from build123d import *

# Parameters (mm, degrees)
BOSS_EXTRUDE1_DEPTH = 2.0574
SKETCH2_R           = 2.54
BOSS_EXTRUDE2_DEPTH = 14.605
FILLET1_R           = 0.635


with BuildPart() as part:
    # Sketch1 → Boss-Extrude1 (new, symmetric)
    with BuildSketch(Plane(origin=(0, 0, 0), x_dir=(1, 0, 0), z_dir=(0, 1, 0))):
        Polygon((-2.7305, -1.57645491), (0, -3.15290982), (2.7305, -1.57645491), (2.7305, 1.57645491), (0, 3.15290982), (-2.7305, 1.57645491), align=None)
    extrude(amount=BOSS_EXTRUDE1_DEPTH, both=True)

    # Sketch2 → Boss-Extrude2 (add)
    with BuildSketch(Plane(origin=(0, 2.0574, 0), x_dir=(1, 0, 0), z_dir=(0, 1, 0))):
        with Locations(Location((0, 0, 0), (0, 0, 90))):
            Circle(SKETCH2_R)
    boss_extrude2 = extrude(amount=BOSS_EXTRUDE2_DEPTH)

    # Mirror1: Boss-Extrude2 across plane
    add(boss_extrude2.mirror(Plane.ZX))

    # Fillet1
    fillet1_edges = [part.edges().sort_by_distance(p)[0] for p in [
        (0, 16.6624, 2.54),
        (0, -16.6624, 2.54),
    ]]
    fillet(fillet1_edges, radius=FILLET1_R)


solid = part.part
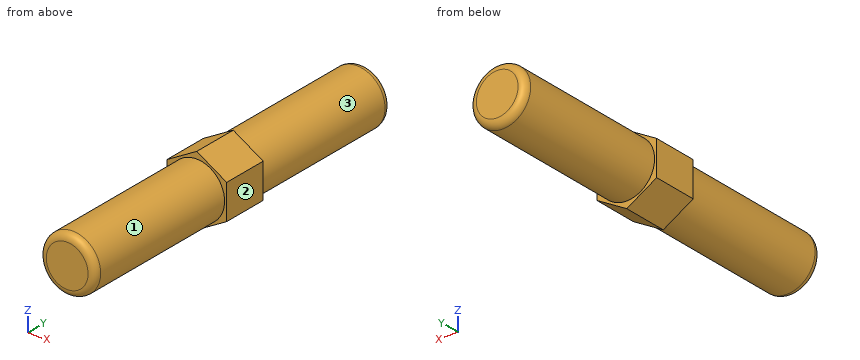
Input: part model. Units: mm. Frame: model coordinates. Face numbers are marked on the shaded views. A direction names the side the tool comes from. Round coordinates to 2 decimals unless told otherwise and drop trailing zeros. Order: outer loops, then holes, each group sorted by start corner. A loop starts at its lowest first (then second) coordinate and runs counter-clockwise, first axis right, second up. Notation, with made-up numbers: (86.5, -31.5) - (120.5, -31.5) arc R30 ccw to (120.5, -9.5) - close; hole circle Ø8 at (69, 30.25). An arc over 180 degrees is marked (long way). Answer as a JSON object with one key per item and string values. Group by question number.
(1) Reachability of the marked faces 1, 2 and 3 from +Z, -Z, +X, -X, +Y, -Y: full face, straight path, thin tool, end or side. Return the list, or none.
(2) Cut plane B-B (y = -8). Return loops of the section in (x, z).
(3) Material intervals for probe 1 along Z at (x, y) = (-0.1, 8.5); probe 2 along Y at (x, z) = (1.9, 0.5); probe 3 along Y at (x, z) = (-0.9, -2.5), sorted ascending. Write a range as from..to.
Here are the results:
{
 "1": {"face 1": "-Y", "face 2": "+Z, -Z, +X, +Y, -Y", "face 3": "+Y"},
 "2": {"outline": "circle Ø5.08 at (0, 0)"},
 "3": {"probe 1": "z = -2.54..2.54", "probe 2": "y = -16.66..16.66", "probe 3": "y = -2.06..2.06"}
}
